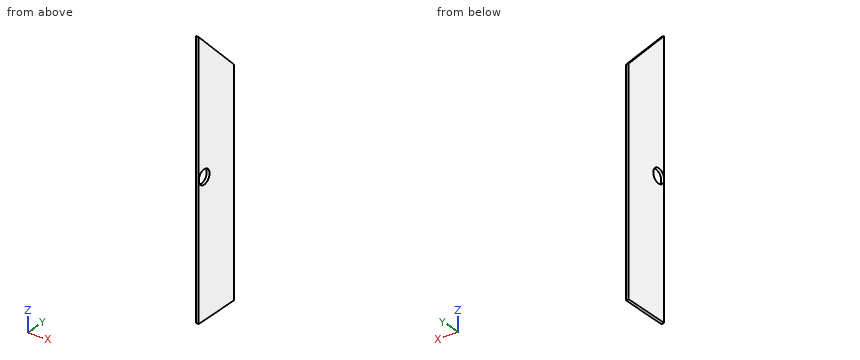
Autodesk Inventor part; units mm, degrees
ref_plane "YZ Plane" through (0, 0, 0) normal (1, 0, 0) x (0, 1, 0)
ref_plane "XZ Plane" through (0, 0, 0) normal (0, 1, 0) x (-1, 0, 0)
ref_plane "XY Plane" through (0, 0, 0) normal (0, 0, 1) x (1, 0, 0)
sketch "Sketch1" plane through (0, 0, 0) normal (1, 0, 0) x (0, 1, 0)
  line L0 (0, 0) -> (0, -280)
  line L1 (0, -280) -> (50, -280)
  line L2 (50, -280) -> (50, -50)
  line L3 (0, 0) -> (0, 0)
  line L4 (50, -50) -> (0, 0)
  dimension "d0" = 280
  dimension "d1" = 50
  dimension "d2" = 90
extrude "Extrusion1" add sketch "Sketch1" along normal blind 3
sketch "Sketch2" plane through (3, 0, 0) normal (1, 0, 0) x (0, 0, -1)
  line L0 (280, 0) -> (280, 50)
  line L1 (280, 50) -> (50, 50)
  line L2 (280, 50) -> (140, 50)
  line L3 (140, 50) -> (140, 7.7)
  point P0 (0, 0)
  dimension "d6" = 140
  dimension "d7" = 42.3
hole "Hole1" at (3, 7.7, -140) direction (-1, 0, 0) diameter 15.2 end through all
sketch "Sketch3" plane through (3, 0, 0) normal (1, 0, 0) x (0, 0, -1)
  point P0 (0, 0)
Read the model definition and answer for the solid it produces. Units are mm, in the model's axes. Give positions to 0.01 mm unless a question says otherwise; leave off trailing zeros. Order: outer loops, then holes, each group sorted by start corner. A loop starts at its lowest first (then second) coordinate and runs counter-clockwise, first axis right, second up. Notation, with made-up numbers: (26.25, 70) -> (83.25, 70) arc R21 cw to (83.25, 88) -> close; hole circle Ø10 at (17.25, 72.5). An arc over 180 degrees is marked (long way). One line per item, written item: value. Start each with the question number.
(1) The part is cut by section D-D (y = 35). Determine the outline of the cut face in (x, z).
(2) The part is cut by section B-B (z = -140). Determine the outline of the cut face in (x, y).
(3) The part is cut by section A-A (y = 7.7). Determine the outline of the cut face in (x, z), and give its area (3 significant figures).
(4) Straight lines are drawn through the part: L1, parallel to Z at x = 1.75, y = 13.5; L2, parallel to Z at x = 0.7, y = 7.7; L3, parallel to Y at x = 0.8, z = -133.5. For each, find the intervals that lie inside material, in ascending order.
(5) The part is cut by section C-C (x = 2.55). Determine the outline of the cut face in (y, z), and give its area (3 significant figures).
(6) Flat-ended cylindrical pins translate along their axes: P1, Ø12, axis at y = 7.7, z = -140, coming from the -X side; P2, Ø1, axis at x = 1, y = 24, coming from the +Z side. Find the tip coordinate at first contact, or state that the pin passes through.
Taken from the geometry:
1. outline: (0, -280) -> (3, -280) -> (3, -35) -> (0, -35) -> close
2. outline: (0, 0) -> (3, 0) -> (3, 0.1) -> (0, 0.1) -> close; (0, 15.3) -> (3, 15.3) -> (3, 50) -> (0, 50) -> close
3. outline: (0, -280) -> (3, -280) -> (3, -147.6) -> (0, -147.6) -> close; (0, -132.4) -> (3, -132.4) -> (3, -7.7) -> (0, -7.7) -> close
3. area: 771 mm^2
4. L1: -280 to -144.91, -135.09 to -13.5
4. L2: -280 to -147.6, -132.4 to -7.7
4. L3: 0 to 3.76, 11.64 to 50
5. outline: (0, -280) -> (50, -280) -> (50, -50) -> (0, 0) -> close; hole circle Ø15.2 at (7.7, -140)
5. area: 12,600 mm^2
6. P1: through
6. P2: z = -23.5
